Read the model definition and answer for the solid it produces. Units are mm, in the model's axes. Round coordinates to 2 decimals unless told otherwise and drop trailing zeros. Write each loop counter-clockwise with the first axis right and the second up, starting at its lowest first coordinate (ties: lowest second). Pieces come first, ordered by that corner, then holes. Notation, with made-up numbers: (-39, 18.25) -> (-14, 18.25) arc R12 cw to (-14, 33.25) -> close; hole circle Ø8 at (45, 54). An arc over 180 degrees is marked (long way). Return JSON: item names as keys, results as strings. Group by question number.
(1) The mould has two halves that part along X. Classify faces 1 (the cylindrical face through (-456.04, -345.52, 1.48)), 2 (the cylindrical face through (-477.517, -394.389, 1.479)), 3 (the flat face through (-463, -375, 0)), 4 (the flat face through (-442.944, -353.576, 1.479)): released by +X, released by -X, zero draft, split by the parting line, or undercut.
(2) A cutting plane is placed at A-A on x = -453. Give the vertices of the cut face in (y, z).
(3) Straight lines are drawn through the part: line 1 (Y direction, x = -452.5, z = 2.1); line 2 (Y direction, x = -477, z = 2.85); line 3 (Y direction, x = -467, z = 2.7). For each, find the intervals that lie inside material, in ascending order.
(4) A cutting plane is placed at B-B on z = 0.8. Give the vertices of the cut face in (x, y).
(5) A cutting plane is placed at D-D on x = -461. Give the vertices of the cut face in (y, z).
(6) A cutting plane is placed at C-C on y = -360. Give the vertices of the cut face in (x, z), then the cut area to 3 significant figures.
Autodesk Inventor part; units mm, degrees
ref_plane "YZ Plane" through (0, 0, 0) normal (1, 0, 0) x (0, 1, 0)
ref_plane "XZ Plane" through (0, 0, 0) normal (0, 1, 0) x (-1, 0, 0)
ref_plane "XY Plane" through (0, 0, 0) normal (0, 0, 1) x (1, 0, 0)
sketch "スケッチ1" plane through (0, 0, 0) normal (0, 0, 1) x (1, 0, 0)
  line L0 (67.5, 17.5) -> (-67.5, 17.5) construction
  line L1 (-67.5, 17.5) -> (-67.5, -17.5) construction
  line L2 (-67.5, -17.5) -> (67.5, -17.5) construction
  line L3 (67.5, -17.5) -> (67.5, 17.5) construction
  line L4 (67.5, 17.5) -> (-67.5, -17.5) construction
  line L5 (-67.5, 17.5) -> (67.5, -17.5) construction
  circle A0 centre (-60, 35) radius 1.6
  circle A1 centre (-70, 35) radius 1.6
  line L6 (-77.5, 27.5) -> (-53, 27.5)
  line L7 (-53, 27.5) -> (-53, 42.5)
  line L8 (-53, 42.5) -> (-80, 42.5) construction
  line L9 (-77.5, 27.5) -> (-77.5, -27.5)
  line L10 (-77.5, -27.5) -> (-53, -27.5)
  line L11 (-53, -27.5) -> (-53, -42.5)
  line L12 (-53, -42.5) -> (-80, -42.5)
  circle A2 centre (-60, -35) radius 1.6
  circle A3 centre (-70, -35) radius 1.6
  circle A4 centre (-80, -35) radius 1.6
  line L13 (124.2308, -31.7536) -> (484.5935, -392.1164)
  line L14 (484.5935, -392.1164) -> (488.7129, -553.575)
  line L15 (-80, 21.2868) -> (-468.838, -367.5512) construction
  line L16 (-468.838, -367.5512) -> (-479.4446, -356.9446) construction
  line L17 (-479.4446, -356.9446) -> (-90.6066, 31.8934) construction
  line L18 (-90.6066, 31.8934) -> (-80, 21.2868) construction
  line L19 (-80, 42.5) -> (-80, 5.3052) construction
  circle A5 centre (-92.3744, 19.519) radius 1.6
  circle A6 centre (-102.981, 8.9124) radius 1.6
  circle A7 centre (-113.5876, -1.6942) radius 1.6
  line L20 (-92.3744, 19.519) -> (-113.5876, -1.6942) construction
  circle A8 centre (-466.4339, -354.5405) radius 1.6
  circle A9 centre (-455.8273, -343.9339) radius 1.6
  line L21 (-388.4374, -772.2067) -> (-358.1265, -754.7067) construction
  line L22 (-358.1265, -754.7067) -> (-425.6265, -637.7933) construction
  line L23 (-455.9374, -655.2933) -> (-358.1265, -754.7067) construction
  line L24 (-388.4374, -772.2067) -> (-425.6265, -637.7933) construction
  line L25 (-455.9374, -655.2933) -> (-388.4374, -772.2067) construction
  line L26 (-425.6265, -637.7933) -> (-455.9374, -655.2933) construction
  line L27 (455.9374, -655.2933) -> (425.6265, -637.7933) construction
  line L28 (425.6265, -637.7933) -> (358.1265, -754.7067) construction
  line L29 (388.4374, -772.2067) -> (425.6265, -637.7933) construction
  line L30 (455.9374, -655.2933) -> (358.1265, -754.7067) construction
  line L31 (388.4374, -772.2067) -> (455.9374, -655.2933) construction
  line L32 (358.1265, -754.7067) -> (388.4374, -772.2067) construction
  line L33 (0, 0) -> (0, -263.4473) construction
  circle A10 centre (80, -35) radius 1.6
  line L34 (67.5, 17.5) -> (67.5, -17.5) construction
  line L35 (77.5, 27.5) -> (53, 27.5)
  line L36 (77.5, 27.5) -> (77.5, -27.5)
  line L37 (77.5, -27.5) -> (53, -27.5)
  circle A11 centre (60, -35) radius 1.6
  circle A12 centre (70, -35) radius 1.6
  line L38 (53, -27.5) -> (53, -42.5)
  line L39 (53, -42.5) -> (80, -42.5)
  circle A13 centre (60, 35) radius 1.6
  circle A14 centre (70, 35) radius 1.6
  line L40 (80, 42.5) -> (80, 5.3052) construction
  line L41 (53, 42.5) -> (80, 42.5)
  line L42 (53, 27.5) -> (53, 42.5)
  line L43 (-392.0976, -785.867) -> (-404.3476, -764.6493)
  line L44 (-388.4374, -772.2067) -> (-358.1265, -754.7067) construction
  line L45 (-392.0976, -785.867) -> (-344.4662, -758.367)
  circle A15 centre (-336.7211, -756.782) radius 1.6
  circle A16 centre (-341.7211, -748.1218) radius 1.6
  line L46 (-343.7259, -729.6493) -> (-330.2259, -753.032)
  circle A17 centre (-346.7211, -739.4615) radius 1.6
  line L47 (-356.7162, -737.1493) -> (-343.7259, -729.6493)
  line L48 (-344.4662, -758.367) -> (-356.7162, -737.1493)
  circle A18 centre (-407.3428, -774.4615) radius 1.6
  circle A19 centre (-402.3428, -783.1218) radius 1.6
  line L49 (-404.3476, -764.6493) -> (-417.338, -772.1493)
  line L50 (-417.338, -772.1493) -> (-403.838, -795.532)
  line L51 (-403.838, -795.532) -> (-371.6264, -776.9346) construction
  line L52 (-425.6265, -637.7933) -> (-455.9374, -655.2933) construction
  line L53 (-409.7162, -645.3507) -> (-396.7259, -637.8507)
  circle A20 centre (-406.7211, -635.5385) radius 1.6
  line L54 (-455.9374, -655.2933) -> (-425.6265, -637.7933) construction
  circle A21 centre (-411.7211, -626.8782) radius 1.6
  line L55 (-469.5976, -651.633) -> (-421.9662, -624.133)
  line L56 (-421.9662, -624.133) -> (-409.7162, -645.3507)
  line L57 (-396.7259, -637.8507) -> (-410.2259, -614.468)
  circle A22 centre (-416.7211, -618.218) radius 1.6
  line L58 (-469.5976, -651.633) -> (-457.3476, -672.8507)
  circle A23 centre (-467.3428, -670.5385) radius 1.6
  circle A24 centre (-472.3428, -661.8782) radius 1.6
  line L59 (-483.838, -656.968) -> (-451.6264, -638.3706) construction
  line L60 (-470.338, -680.3507) -> (-483.838, -656.968)
  line L61 (-457.3476, -672.8507) -> (-470.338, -680.3507)
  line L62 (469.5976, -651.633) -> (457.3476, -672.8507)
  line L63 (455.9374, -655.2933) -> (425.6265, -637.7933) construction
  line L64 (469.5976, -651.633) -> (421.9662, -624.133)
  circle A25 centre (416.7211, -618.218) radius 1.6
  circle A26 centre (411.7211, -626.8782) radius 1.6
  line L65 (396.7259, -637.8507) -> (410.2259, -614.468)
  circle A27 centre (406.7211, -635.5385) radius 1.6
  line L66 (409.7162, -645.3507) -> (396.7259, -637.8507)
  line L67 (421.9662, -624.133) -> (409.7162, -645.3507)
  circle A28 centre (467.3428, -670.5385) radius 1.6
  circle A29 centre (472.3428, -661.8782) radius 1.6
  line L68 (457.3476, -672.8507) -> (470.338, -680.3507)
  line L69 (470.338, -680.3507) -> (483.838, -656.968)
  line L70 (483.838, -656.968) -> (451.6264, -638.3706) construction
  line L71 (358.1265, -754.7067) -> (388.4374, -772.2067) construction
  line L72 (356.7162, -737.1493) -> (343.7259, -729.6493)
  circle A30 centre (346.7211, -739.4615) radius 1.6
  line L73 (388.4374, -772.2067) -> (358.1265, -754.7067) construction
  circle A31 centre (341.7211, -748.1218) radius 1.6
  line L74 (392.0976, -785.867) -> (344.4662, -758.367)
  line L75 (344.4662, -758.367) -> (356.7162, -737.1493)
  line L76 (343.7259, -729.6493) -> (330.2259, -753.032)
  circle A32 centre (336.7211, -756.782) radius 1.6
  line L77 (392.0976, -785.867) -> (404.3476, -764.6493)
  circle A33 centre (407.3428, -774.4615) radius 1.6
  circle A34 centre (402.3428, -783.1218) radius 1.6
  line L78 (403.838, -795.532) -> (371.6264, -776.9346) construction
  line L79 (417.338, -772.1493) -> (403.838, -795.532)
  line L80 (404.3476, -764.6493) -> (417.338, -772.1493)
  line L81 (-483.838, -367.5512) -> (-468.838, -367.5512) construction
  line L82 (-468.838, -367.5512) -> (-468.838, -648.3077) construction
  line L83 (-468.838, -648.3077) -> (-483.838, -648.3077)
  line L84 (-483.838, -648.3077) -> (-483.838, -367.5512) construction
  line L85 (-283.2277, -604.4352) -> (-262.2277, -640.8083) construction
  line L86 (345.2492, -497.0108) -> (305.7786, -565.3759) construction
  line L87 (265.1134, -631.6538) -> (-234.8866, -631.6538) construction
  line L88 (-234.8866, -631.6538) -> (-234.8866, -1131.6538) construction
  line L89 (-234.8866, -1131.6538) -> (265.1134, -1131.6538) construction
  line L90 (265.1134, -1131.6538) -> (265.1134, -631.6538) construction
  line L91 (265.1134, -631.6538) -> (-234.8866, -1131.6538) construction
  line L92 (-234.8866, -631.6538) -> (265.1134, -1131.6538) construction
  line L93 (-12.841, -157.5) -> (15.1134, -157.5) construction
  circle A35 centre (1.1362, -409.4569) radius 212.5 construction
  line L94 (501.1362, 53.616) -> (-498.8638, 53.616) construction
  line L95 (-498.8638, 53.616) -> (-498.8638, -946.384) construction
  line L96 (-498.8638, -946.384) -> (501.1362, -946.384) construction
  line L97 (501.1362, -946.384) -> (501.1362, 53.616) construction
  line L98 (501.1362, 53.616) -> (-498.8638, -946.384) construction
  line L99 (-498.8638, 53.616) -> (501.1362, -946.384) construction
  circle A36 centre (1.1362, -409.4569) radius 250 construction
  line L100 (-80, 42.5) -> (-90.6066, 31.8934) construction
  line L101 (-80, 42.5) -> (-118.8909, 3.6091)
  line L102 (-118.8909, -6.9975) -> (-113.5876, -12.3008)
  line L103 (-113.5876, -12.3008) -> (-85.2767, -40.3298)
  arc A37 (-118.8909, 3.6091) -> (-118.8909, -6.9975) centre (-113.5876, -1.6942) ccw
  arc A38 (-85.2767, -40.3298) -> (-80, -42.5) centre (-80, -35) ccw
  line L104 (-80, 42.5) -> (-53, 42.5)
  line L105 (-466.4339, -354.5405) -> (-455.8273, -343.9339) construction
  circle A39 centre (-476.338, -638.3077) radius 1.6
  circle A40 centre (-476.338, -623.3077) radius 1.6
  circle A41 centre (-476.338, -378.3077) radius 1.6
  circle A42 centre (-476.338, -393.3077) radius 1.6
  line L106 (-454.0595, -331.5595) -> (-443.4529, -342.1661)
  line L107 (-468.838, -403.3077) -> (-475.5897, -403.3077)
  line L108 (-483.838, -403.3077) -> (-483.838, -367.5512)
  line L109 (-454.0595, -331.5595) -> (-479.4446, -356.9446)
  arc A43 (-479.4446, -356.9446) -> (-483.838, -367.5512) centre (-468.838, -367.5512) ccw
  arc A44 (-475.5897, -403.3077) -> (-477.0864, -403.3077) centre (-476.338, -404.6077) ccw
  line L110 (-475.5897, -403.3077) -> (-477.0864, -403.3077) construction
  line L111 (-477.0864, -403.3077) -> (-483.838, -403.3077)
  circle A45 centre (-452.5, -386.0383) radius 1.6
  circle A46 centre (-452.5, -371.0383) radius 1.6
  circle A47 centre (-262.5, -371.0383) radius 1.6 construction
  line L112 (-462.5, -393.5383) -> (-274.6134, -393.5383) construction
  line L113 (-274.6134, -393.5383) -> (-274.6134, -363.5383) construction
  line L114 (-274.6134, -363.5383) -> (-462.5, -363.5383) construction
  line L115 (-462.5, -363.5383) -> (-462.5, -393.5383) construction
  line L116 (-442.5, -393.5383) -> (-442.5, -363.5383)
  line L117 (-468.838, -403.3077) -> (-442.5, -393.5383)
  line L118 (-442.5, -363.5383) -> (-443.4529, -342.1661)
  point P0 (0, -470)
  point P1 (-102.981, 8.9124)
  point P2 (-77.5, 0)
  point P3 (-407.0319, -705)
  point P4 (-407.0319, -705)
  point P5 (407.0319, -705)
  point P6 (407.0319, -705)
  point P7 (77.5, 0)
  point P8 (-368.2819, -772.117)
  point P9 (-385.4668, -784.9254)
  point P10 (-445.7819, -637.883)
  point P11 (445.7819, -637.883)
  point P12 (465.4668, -646.3614)
  point P13 (368.2819, -772.117)
  point P14 (15.1134, -881.6538)
  point P15 (1.1362, -446.384)
  point P16 (-124.1942, -1.6942)
  point P17 (-476.338, -648.3077)
  point P18 (-476.338, -367.5512)
  dimension "d4" = 135
  dimension "d5" = 35
  dimension "d6" = 3.2
  dimension "d7" = 3.2
  dimension "d8" = 10
  dimension "d9" = 15
  dimension "d10" = 10
  dimension "d11" = 7.5
  dimension "d12" = 7
  dimension "d13" = 70
  dimension "d14" = 3.2
  dimension "d15" = 3.2
  dimension "d16" = 3.2
  dimension "d17" = 10
  dimension "d18" = 10
  dimension "d19" = 7
  dimension "d20" = 15
  dimension "d21" = 7.5
  dimension "d22" = 10
  dimension "d23" = 10
  dimension "d24" = 135
  dimension "d25" = 15
  dimension "d26" = 10
  dimension "d27" = 3.2
  dimension "d28" = 3.2
  dimension "d29" = 3.2
  dimension "d30" = 10
  dimension "d31" = 15
  dimension "d32" = 15
  dimension "d33" = 7.5
  dimension "d34" = 45
  dimension "d35" = 3.2
  dimension "d36" = 3.2
  dimension "d37" = 360
  dimension "d38" = 360
  dimension "d39" = 470
  dimension "d40" = 15
  dimension "d41" = 200
  dimension "d42" = 200
  dimension "d43" = 500
  dimension "d44" = 500
  dimension "d45" = 200
  dimension "d46" = 425
  dimension "d47" = 1000
  dimension "d48" = 1000
  dimension "d49" = 42
  dimension "d50" = 500
  dimension "d51" = 7.5
  dimension "d52" = 7.5
  dimension "d53" = 7.5
  dimension "d54" = 484
  dimension "d55" = 15
  dimension "d56" = 3.2
  dimension "d57" = 3.2
  dimension "d58" = 10
  dimension "d59" = 15
  dimension "d60" = 3.2
  dimension "d61" = 3.2
  dimension "d62" = 15
  dimension "d63" = 230
  dimension "d64" = 10
  dimension "d65" = 10
  dimension "d69" = 3
  dimension "d70" = 1.3
extrude "押し出し1" add sketch "スケッチ1" along normal blind 3 contours L106 L118 L116 L117 L107 A44 L111 L108 A43 L109
fillet "フィレット2" radius 3 6 edges at (-483.838, -403.3077, 1.5) (-468.838, -403.3077, 1.5) (-442.5, -393.5383, 1.5) (-442.5, -363.5383, 1.5) (-443.4529, -342.1661, 1.5) (-454.0595, -331.5595, 1.5)
properties part number "オムニ_固定具1" material "アルミニウム 6061"
Checks:
{
 "1": {"face 1": "undercut", "face 2": "undercut", "face 3": "zero draft", "face 4": "released by +X"},
 "2": {"outline": "(-397.43, 0) -> (-387.56, 0) -> (-387.56, 3) -> (-397.43, 3) -> close; (-384.52, 0) -> (-372.56, 0) -> (-372.56, 3) -> (-384.52, 3) -> close; (-369.52, 0) -> (-333, 0) -> (-333, 3) -> (-369.52, 3) -> close"},
 "3": {"line 1": "y = -397.25 to -387.64, -384.44 to -372.64, -369.44 to -333.24", "line 2": "y = -403.26 to -394.76, -391.85 to -379.76, -376.85 to -354.5", "line 3": "y = -402.63 to -356.04, -353.04 to -344.5"},
 "4": {"outline": "(-483.84, -400.31) arc R3 ccw to (-480.84, -403.31) -> (-477.09, -403.31) arc R1.5 cw to (-475.59, -403.31) -> (-469.38, -403.31) arc R3 ccw to (-468.33, -403.12) -> (-444.46, -394.26) arc R3 ccw to (-442.5, -391.45) -> (-442.5, -363.54) -> (-443.4, -343.33) arc R3 ccw to (-444.28, -341.34) -> (-451.94, -333.68) arc R3 ccw to (-456.18, -333.68) -> (-479.44, -356.94) arc R15 ccw to (-483.84, -367.55) -> close; hole circle Ø3.2 at (-476.34, -393.31); hole circle Ø3.2 at (-476.34, -378.31); hole circle Ø3.2 at (-466.43, -354.54); hole circle Ø3.2 at (-455.83, -343.93); hole circle Ø3.2 at (-452.5, -386.04); hole circle Ø3.2 at (-452.5, -371.04)"},
 "5": {"outline": "(-400.4, 0) -> (-338.5, 0) -> (-338.5, 3) -> (-400.4, 3) -> close"},
 "6": {"outline": "(-481.8, 0) -> (-442.66, 0) -> (-442.66, 3) -> (-481.8, 3) -> close", "area": "117 mm^2"}
}
